```python
from build123d import *


with BuildPart() as f1:
    # F0 (on Front) → F1 (revolve)
    with BuildSketch(Plane.XZ):
        with BuildLine():
            Line((-7.62, -63.5), (0, -63.5))
            Line((0, -63.5), (0, 0))
            Line((0, 0), (-1.27, -2.199705))
            Line((-1.27, -2.199705), (-0.830059, -2.453705))
            Line((-0.830059, -2.453705), (-3.015385, -5.574674))
            Line((-3.015385, -5.574674), (-2.183127, -6.157427))
            Line((-2.183127, -6.157427), (-5.448488, -10.048933))
            ThreePointArc((-5.448488, -10.048933), (-3.707992, -11.330441), (-1.638488, -11.953933))
            Line((-1.638488, -11.953933), (-1.638488, -14.493933))
            Line((-1.638488, -14.493933), (-7.330122, -17.78))
            ThreePointArc((-7.330122, -17.78), (-4.934768, -27.976239), (-7.62, -38.1))
            ThreePointArc((-7.62, -38.1), (-11.750387, -50.8), (-7.62, -63.5))
        make_face()
    revolve(axis=Axis((0, 0, -31.75), (0, 0, -1)))


solid = f1.part
```
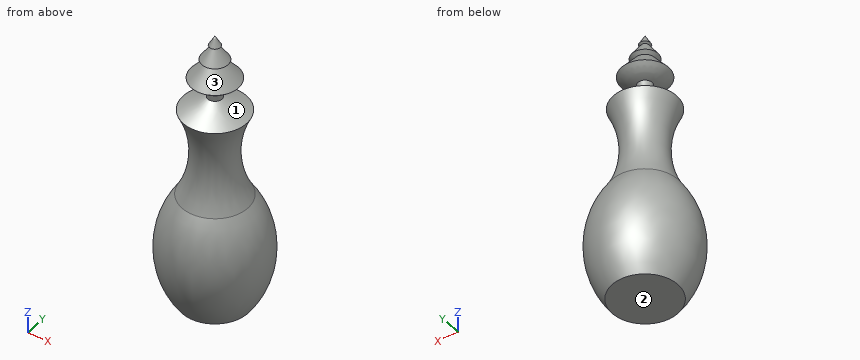
Build history of the part. All positions in model axes, mm. Face numbers are marked on the shaded views. Give positions to 0.01 mm unless a question says otherwise; leave off trailing zeros. Order: outer loops, then holes, each group sorted by start corner. A loop starts at its lowest first (then second) coordinate and runs counter-clockwise, first axis right, second up. Notation, with made-up numbers: M -21.75,-19.75 L 37.25,-19.75 A16 ccw 37.25,-4.75 Z; hole C -24.75,25 d2. An arc over 180 degrees is marked long. Write item = value, one per line. Start each with the question number.
(1) Slice it at A-A on z = -4.5. Write the cut outline in (x, y), plus the area to 3 significant figures.
(2) Slice it at B-B on z = -22. Write the cut outline in (x, y).
(3) Probe L1, parallel to Z at x = -5.5, y = 4.25; L2, parallel to Z at x = -6.75, y = -0.5; L3, parallel to X at y = -1.75, z = -57. List the from-to ranges inside material, lowest first. Write a range as [from, to].
(4) Two-plate mould, pull along Z, no slides. Class the marked faces 1, 2 and 3: released by +Z, released by -Z, zero draft, split by the parting line, or undercut.
(5) Pin check, flat tips, straight feed: pin 1 Ø6 at (y, z) = (-4, -48.5) entering from -X; pin 2 Ø3 at (x, y) = (7.5, -1.5) entering from -Z; pin 3 Ø5 at (x, z) = (3, -15) entering from -Y; pin 4 Ø4 at (y, z) = (-4.5, -8.5) entering from -X. Stop position of each tip, or through.
Responses:
q1.outline = C 0,0 d4.53
q1.area = 16.1 mm2
q2.outline = C 0,0 d11.38
q3.L1 = [-63.5, -36.78], [-18.55, -17.56]
q3.L2 = [-63.5, -36.38], [-18.96, -17.46]
q3.L3 = [-10.7, 10.7]
q4.face_1 = undercut
q4.face_2 = released by -Z
q4.face_3 = undercut
q5.pin_1 = -11.66
q5.pin_2 = -63.5
q5.pin_3 = -6.28
q5.pin_4 = -4.38
